CAD build for the part. Positions are in the model's coordinates, mm. A direction names the side the tool comes from. Give positions to 0.01 mm unless a question says otherwise; leave off trailing zeros. Write each loop counter-clockwise with the first axis right and the second up, starting at its lowest first coordinate (ties: lowest second). Pieces come first, ordered by that corner, then holes. Notation, with made-up numbers: (-20.75, 31) -> (4.25, 31) arc R28 ccw to (4.25, 53) -> close; hole circle Ø2 at (34, 43). An arc over 180 degrees is marked (long way). Answer as a JSON object with one key per item and string values.
Autodesk Inventor part; units mm, degrees
ref_plane "YZ Plane" through (0, 0, 0) normal (1, 0, 0) x (0, 1, 0)
ref_plane "XZ Plane" through (0, 0, 0) normal (0, 1, 0) x (-1, 0, 0)
ref_plane "XY Plane" through (0, 0, 0) normal (0, 0, 1) x (1, 0, 0)
sketch "Sketch1" plane through (0, 0, 0) normal (0, 0, 1) x (1, 0, 0)
  arc A0 (-12.6, 10.95) -> (-15.1, 8.45) centre (-12.6, 8.45) ccw
  line L0 (-15.1, 8.45) -> (-15.1, -8.45)
  arc A1 (-15.1, -8.45) -> (-12.6, -10.95) centre (-12.6, -8.45) ccw
  line L1 (-12.6, -10.95) -> (12.6, -10.95)
  arc A2 (12.6, -10.95) -> (15.1, -8.45) centre (12.6, -8.45) ccw
  line L2 (15.1, -8.45) -> (15.1, 8.45)
  arc A3 (15.1, 8.45) -> (12.6, 10.95) centre (12.6, 8.45) ccw
  line L3 (12.6, 10.95) -> (-12.6, 10.95)
  circle A4 centre (11.825, 7.675) radius 1.575
  circle A5 centre (11.825, -7.675) radius 1.575
  line L4 (15.7, 8.45) -> (15.7, -8.45)
  arc A6 (12.6, -11.55) -> (15.7, -8.45) centre (12.6, -8.45) ccw
  line L5 (12.6, -11.55) -> (-12.6, -11.55)
  arc A7 (-15.7, -8.45) -> (-12.6, -11.55) centre (-12.6, -8.45) ccw
  line L6 (-15.7, -8.45) -> (-15.7, 8.45)
  arc A8 (-12.6, 11.55) -> (-15.7, 8.45) centre (-12.6, 8.45) ccw
  line L7 (-12.6, 11.55) -> (12.6, 11.55)
  arc A9 (15.7, 8.45) -> (12.6, 11.55) centre (12.6, 8.45) ccw
  line L8 (19.7, -8.45) -> (19.7, 8.45)
  arc A10 (19.7, 8.45) -> (12.6, 15.55) centre (12.6, 8.45) ccw
  line L9 (12.6, 15.55) -> (-12.6, 15.55)
  arc A11 (-12.6, 15.55) -> (-19.7, 8.45) centre (-12.6, 8.45) ccw
  line L10 (-19.7, 8.45) -> (-19.7, -8.45)
  arc A12 (-19.7, -8.45) -> (-12.6, -15.55) centre (-12.6, -8.45) ccw
  line L11 (-12.6, -15.55) -> (12.6, -15.55)
  arc A13 (12.6, -15.55) -> (19.7, -8.45) centre (12.6, -8.45) ccw
  point P0 (0, 0)
  dimension "d0" = 0.6
  dimension "d1" = 4
extrude "Extrusion1" add sketch "Sketch1" along normal blind 5 contours L3 A3 L2 A2 L1 A1 L0 A0 | A4 | A5 | L4 A6 L5 A7 L6 A8 L7 A9 | A13 L11 A12 L10 A11 L9 A10 L8
sketch "Sketch2" plane through (0, 0, 0) normal (0, 0, -1) x (-1, 0, 0)
  line L0 (12.6, 11.55) -> (-12.6, 11.55)
  arc A0 (15.7, 8.45) -> (12.6, 11.55) centre (12.6, 8.45) ccw
  line L1 (15.7, -8.45) -> (15.7, 8.45)
  arc A1 (12.6, -11.55) -> (15.7, -8.45) centre (12.6, -8.45) ccw
  line L2 (12.6, -10.95) -> (-12.6, -10.95)
  arc A2 (-15.7, -8.45) -> (-12.6, -11.55) centre (-12.6, -8.45) ccw
  line L3 (-15.7, 8.45) -> (-15.7, -8.45)
  arc A3 (-12.6, 11.55) -> (-15.7, 8.45) centre (-12.6, 8.45) ccw
  arc A4 (-12.6, 15.55) -> (-19.7, 8.45) centre (-12.6, 8.45) ccw
  line L4 (-19.7, -8.45) -> (-19.7, 8.45)
  arc A5 (-19.7, -8.45) -> (-12.6, -15.55) centre (-12.6, -8.45) ccw
  line L5 (12.6, -15.55) -> (-12.6, -15.55)
  arc A6 (12.6, -15.55) -> (19.7, -8.45) centre (12.6, -8.45) ccw
  line L6 (19.7, 8.45) -> (19.7, -8.45)
  arc A7 (19.7, 8.45) -> (12.6, 15.55) centre (12.6, 8.45) ccw
  line L7 (-12.6, 15.55) -> (12.6, 15.55)
  line L8 (7.1, -5) -> (15.1, -5)
  line L9 (15.1, -5) -> (15.1, 5)
  line L10 (15.1, 5) -> (7.1, 5)
  line L11 (7.1, 5) -> (7.1, -5)
  line L12 (15.7, 7) -> (19.7, 7)
  line L13 (19.7, 7) -> (19.7, -7)
  line L14 (19.7, -7) -> (15.7, -7)
  line L15 (15.7, -7) -> (15.7, 7)
  line L16 (15.7, 7) -> (19.7, -7) construction
  line L17 (19.7, 7) -> (15.7, -7) construction
  line L18 (-12.6, -11.55) -> (12.6, -11.55)
  point P0 (0, 0)
  point P1 (17.7, 0)
  point P2 (19.7, 0)
  point P3 (17.7, 7)
  dimension "d4" = 2
extrude "Extrusion2" add sketch "Sketch2" along normal blind 9.8 contours L0 A3 L3 A2 L18 A1 L1 L14 L6 A6 L5 A5 L4 A4 L7 A7 L12 A0
sketch "Sketch3" plane through (0, 0, 0) normal (0, 0, -1) x (-1, 0, 0)
  circle A0 centre (-11.825, -7.675) radius 1.575
  circle A1 centre (-11.825, 7.675) radius 1.575
  circle A2 centre (-11.825, -7.675) radius 1.2
  circle A3 centre (-11.825, 7.675) radius 1.2
  point P0 (0, 0)
  dimension "d7" = 3.15
  dimension "d8" = 2.4
  dimension "d9" = 2.4
extrude "Extrusion3" cut sketch "Sketch3" against normal blind 3 contours A2 | A3
sketch "Sketch4" plane through (0, 0, 5) normal (0, 0, 1) x (1, 0, 0)
  arc A0 (19.7, 8.45) -> (12.6, 15.55) centre (12.6, 8.45) ccw
  line L0 (12.6, 15.55) -> (-12.6, 15.55)
  arc A1 (-12.6, 15.55) -> (-19.7, 8.45) centre (-12.6, 8.45) ccw
  line L1 (-19.7, 8.45) -> (-19.7, -8.45)
  arc A2 (-19.7, -8.45) -> (-12.6, -15.55) centre (-12.6, -8.45) ccw
  line L2 (-12.6, -15.55) -> (12.6, -15.55)
  arc A3 (12.6, -15.55) -> (19.7, -8.45) centre (12.6, -8.45) ccw
  line L3 (19.7, -8.45) -> (19.7, 8.45)
  line L4 (-2.6, -15.55) -> (-12.6, -15.55)
  line L5 (-12.6, -15.55) -> (-12.6, -25.55)
  line L6 (-12.6, -25.55) -> (-2.6, -25.55)
  line L7 (-2.6, -25.55) -> (-2.6, -15.55)
  line L8 (-2.6, -15.55) -> (-12.6, -25.55) construction
  line L9 (-12.6, -15.55) -> (-2.6, -25.55) construction
  line L10 (-12.6, -15.55) -> (12.6, -15.55)
  line L11 (19.7, 0) -> (-19.7, 0)
  line L12 (0, 15.55) -> (0, -15.55)
  line L13 (-2.6, 15.55) -> (-12.6, 15.55)
  line L14 (-12.6, 15.55) -> (-12.6, 25.55)
  line L15 (-12.6, 25.55) -> (-2.6, 25.55)
  line L16 (-2.6, 25.55) -> (-2.6, 15.55)
  line L17 (-2.6, 15.55) -> (-12.6, 25.55) construction
  line L18 (-12.6, 15.55) -> (-2.6, 25.55) construction
  arc A4 (19.7, 8.45) -> (12.6, 15.55) centre (12.6, 8.45) ccw
  line L19 (2.6, 15.55) -> (12.6, 15.55)
  line L20 (2.6, 25.55) -> (2.6, 15.55)
  line L21 (2.6, 15.55) -> (12.6, 25.55) construction
  line L22 (12.6, 25.55) -> (2.6, 25.55)
  line L23 (12.6, 15.55) -> (2.6, 25.55) construction
  line L24 (12.6, 15.55) -> (12.6, 25.55)
  line L25 (2.6, -15.55) -> (12.6, -15.55)
  line L26 (2.6, -25.55) -> (2.6, -15.55)
  line L27 (2.6, -15.55) -> (12.6, -25.55) construction
  line L28 (12.6, -15.55) -> (2.6, -25.55) construction
  line L29 (12.6, -15.55) -> (12.6, -25.55)
  line L30 (12.6, -25.55) -> (2.6, -25.55)
  point P0 (0, 0)
  point P1 (-7.6, -20.55)
  point P2 (-7.6, 20.55)
  point P3 (7.6, 20.55)
  point P4 (2.6, 15.55)
  point P5 (-2.6, 15.55)
  point P6 (7.6, -20.55)
  point P7 (2.6, -15.55)
  dimension "d12" = 10
  dimension "d13" = 10
extrude "Extrusion4" add sketch "Sketch4" against normal blind 11 contours L0 L20 L22 L24 | L29 L30 L26 L2
sketch "Sketch5" plane through (0, 0, -6) normal (0, 0, -1) x (-1, 0, 0)
  line L0 (-12.6, -15.55) -> (-2.6, -15.55)
  line L1 (5.6, -22.55) -> (12.6, -15.55)
  line L2 (4.1, -17.05) -> (11.1, -24.05)
  line L3 (12.6, -11.55) -> (-12.6, -11.55)
  arc A0 (-15.7, -8.45) -> (-12.6, -11.55) centre (-12.6, -8.45) ccw
  line L4 (-15.7, -8.45) -> (-15.7, 8.45)
  arc A1 (-12.6, 11.55) -> (-15.7, 8.45) centre (-12.6, 8.45) ccw
  line L5 (-12.6, 11.55) -> (12.6, 11.55)
  arc A2 (15.7, 8.45) -> (12.6, 11.55) centre (12.6, 8.45) ccw
  line L6 (15.7, 8.45) -> (15.7, 7)
  line L7 (15.7, 7) -> (19.7, 7)
  line L8 (19.7, 7) -> (19.7, 8.45)
  arc A3 (19.7, 8.45) -> (12.6, 15.55) centre (12.6, 8.45) ccw
  line L9 (12.6, 15.55) -> (-12.6, 15.55)
  arc A4 (-12.6, 15.55) -> (-19.7, 8.45) centre (-12.6, 8.45) ccw
  line L10 (-19.7, 8.45) -> (-19.7, -8.45)
  arc A5 (-19.7, -8.45) -> (-12.6, -15.55) centre (-12.6, -8.45) ccw
  line L11 (-12.6, -15.55) -> (12.6, -15.55)
  arc A6 (12.6, -15.55) -> (19.7, -8.45) centre (12.6, -8.45) ccw
  line L12 (19.7, -8.45) -> (19.7, -7)
  line L13 (19.7, -7) -> (15.7, -7)
  line L14 (15.7, -7) -> (15.7, -8.45)
  arc A7 (12.6, -11.55) -> (15.7, -8.45) centre (12.6, -8.45) ccw
  circle A8 centre (-11.825, 7.675) radius 1.2
  circle A9 centre (-11.825, -7.675) radius 1.2
  line L15 (19.7, 7) -> (15.7, 7)
  line L16 (15.7, 7) -> (15.7, 8.45)
  arc A10 (15.7, 8.45) -> (12.6, 11.55) centre (12.6, 8.45) ccw
  line L17 (12.6, 11.55) -> (-12.6, 11.55)
  arc A11 (-12.6, 11.55) -> (-15.7, 8.45) centre (-12.6, 8.45) ccw
  line L18 (-15.7, 8.45) -> (-15.7, -8.45)
  arc A12 (-15.7, -8.45) -> (-12.6, -11.55) centre (-12.6, -8.45) ccw
  line L19 (-12.6, -11.55) -> (12.6, -11.55)
  arc A13 (12.6, -11.55) -> (15.7, -8.45) centre (12.6, -8.45) ccw
  line L20 (15.7, -8.45) -> (15.7, -7)
  line L21 (15.7, -7) -> (19.7, -7)
  line L22 (19.7, 7) -> (19.7, -7)
  line L23 (19.7, 0) -> (-19.7, 0)
  line L24 (0, -15.55) -> (0, 15.55)
  line L25 (-12.6, -15.55) -> (-12.6, -25.55)
  line L26 (-12.6, -25.55) -> (-2.6, -25.55)
  line L27 (-2.6, -25.55) -> (-2.6, -15.55)
  point P0 (0, 0)
  point P1 (7.6, -20.55)
  point P2 (7.6, 20.55)
  point P3 (-7.6, 20.55)
  point P4 (-7.6, -20.55)
hole "Hole1" at (7.6, 20.55, -6) at (7.6, -20.55, -6) direction (0, 0, 1) diameter 4.5 end through all
fillet "Fillet1" radius 1 2 edges at (12.6, -15.55, -0.5) (12.6, 15.55, -0.5)
fillet "Fillet2" radius 1 6 edges at (2.6, -15.55, -0.5) (2.6, 15.55, -0.5) (12.6, 25.55, -0.5) (2.6, 25.55, -0.5) (2.6, -25.55, -0.5) (12.6, -25.55, -0.5)
sketch "Sketch6" plane through (0, 0, -9.8) normal (0, 0, -1) x (-1, 0, 0)
  line L0 (12.6, -11.55) -> (-12.6, -11.55)
  arc A0 (-15.7, -8.45) -> (-12.6, -11.55) centre (-12.6, -8.45) ccw
  line L1 (-15.7, -8.45) -> (-15.7, 8.45)
  arc A1 (-12.6, 11.55) -> (-15.7, 8.45) centre (-12.6, 8.45) ccw
  line L2 (-12.6, 11.55) -> (12.6, 11.55)
  arc A2 (15.7, 8.45) -> (12.6, 11.55) centre (12.6, 8.45) ccw
  line L3 (15.7, 8.45) -> (15.7, 7)
  line L4 (15.7, 7) -> (19.7, 7)
  line L5 (19.7, 7) -> (19.7, 8.45)
  arc A3 (19.7, 8.45) -> (12.6, 15.55) centre (12.6, 8.45) ccw
  line L6 (12.6, 15.55) -> (-13.2535, 15.55)
  arc A4 (-13.4765, 15.4957) -> (-13.2535, 15.55) centre (-13.6, 16.488) ccw
  arc A5 (-13.4765, 15.4957) -> (-19.7, 8.45) centre (-12.6, 8.45) ccw
  line L7 (-19.7, 8.45) -> (-19.7, -8.45)
  arc A6 (-19.7, -8.45) -> (-13.4765, -15.4957) centre (-12.6, -8.45) ccw
  arc A7 (-13.2535, -15.55) -> (-13.4765, -15.4957) centre (-13.6, -16.488) ccw
  line L8 (-13.2535, -15.55) -> (12.6, -15.55)
  arc A8 (12.6, -15.55) -> (19.7, -8.45) centre (12.6, -8.45) ccw
  line L9 (19.7, -8.45) -> (19.7, -7)
  line L10 (19.7, -7) -> (15.7, -7)
  line L11 (15.7, -7) -> (15.7, -8.45)
  arc A9 (12.6, -11.55) -> (15.7, -8.45) centre (12.6, -8.45) ccw
  arc A10 (-12.6, 15.55) -> (-19.7, 8.45) centre (-12.6, 8.45) ccw
  arc A11 (-19.7, -8.45) -> (-12.6, -15.55) centre (-12.6, -8.45) ccw
  point P0 (0, 0)
extrude "Extrusion5" cut sketch "Sketch6" against normal up to surface (3.8 mm away) contours L8 A7 A11 | A4 L6 A10
equation "\"d9\" = d8"
properties part number "PrzyciskSTOP_1_3DPrint"
1) Wall check: probe 1 along Y at (x, z) = (7.6, 3.25); probe 2 along Y at (x, z) = (7.6, -1.5); probe 3 along X at (y, z) = (-20.55, -1.25). Give the ranges that are in metal, low to high.
Model answer:
{"probe 1": "y = -25.55 to -22.8, -18.3 to 18.3, 22.8 to 25.55", "probe 2": "y = -25.55 to -22.8, -18.3 to -11.55, 11.55 to 18.3, 22.8 to 25.55", "probe 3": "x = 2.6 to 5.35, 9.85 to 12.6"}
2) Pin check, flat tips, straight feed: pin 1 (5 mm diameter, centred on x = -5.5, y = 20, fed in from -Z); pin 2 (3 mm diameter, centred on y = 12, z = 3, fed in from -X); pin 3 (1.5 mm diameter, centred on x = -12.5, y = 5.5, fed in from -Z); pin 4 (3 mm diameter, centred on y = -17.5, z = -1.5, fed in from -X). Stop position of each tip, or through.
Model answer:
{"pin 1": "passes through", "pin 2": "stops at x = -19.4", "pin 3": "stops at z = 0", "pin 4": "stops at x = 2.44"}
3) Mould opens along Y. For faces 1 (the flat face through (-3, 15.55, -4)), 2 (the flat face through (2.6, 21, 0)), 3 (the flat face through (-15.7, 8, -5)) say: released by +Y, released by -Y, zero draft, split by the parting line, or undercut.
Model answer:
{"face 1": "released by +Y", "face 2": "zero draft", "face 3": "undercut"}
4) Slice it at C-C (x = -1). List the corners of the cut face in (y, z).
Model answer:
{"outline": "(-15.55, -9.8) -> (-11.55, -9.8) -> (-11.55, 0) -> (11.55, 0) -> (11.55, -9.8) -> (15.55, -9.8) -> (15.55, 5) -> (-15.55, 5) -> close"}
5) Slice it at B-B (y = -20.55). List the corners of the cut face in (x, z), then the cut area to 3 significant figures.
Model answer:
{"outline": "(2.6, -6) -> (5.35, -6) -> (5.35, 5) -> (2.6, 5) -> close; (9.85, -6) -> (12.6, -6) -> (12.6, 5) -> (9.85, 5) -> close", "area": "60.5 mm2"}
6) Slice it at D-D (z = 1). List the corners of the cut face in (x, y) (3 decimals).
Model answer:
{"outline": "(-19.7, -8.45) arc R7.1 ccw to (-12.6, -15.55) -> (1.6, -15.55) arc R1 cw to (2.6, -16.55) -> (2.6, -24.55) arc R1 ccw to (3.6, -25.55) -> (11.6, -25.55) arc R1 ccw to (12.6, -24.55) -> (12.6, -16.488) arc R1 cw to (13.477, -15.496) arc R7.1 ccw to (19.7, -8.45) -> (19.7, 8.45) arc R7.1 ccw to (13.477, 15.496) arc R1 cw to (12.6, 16.488) -> (12.6, 24.55) arc R1 ccw to (11.6, 25.55) -> (3.6, 25.55) arc R1 ccw to (2.6, 24.55) -> (2.6, 16.55) arc R1 cw to (1.6, 15.55) -> (-12.6, 15.55) arc R7.1 ccw to (-19.7, 8.45) -> close; hole circle Ø4.5 at (7.6, -20.55); hole circle Ø4.5 at (7.6, 20.55); hole circle Ø2.4 at (11.825, -7.675); hole circle Ø2.4 at (11.825, 7.675)"}
7) Slice it at A-A (x = 7.6). List the corners of the cut face in (y, z).
Model answer:
{"outline": "(-25.55, -6) -> (-22.8, -6) -> (-22.8, 5) -> (-25.55, 5) -> close; (-18.3, -6) -> (-15.55, -6) -> (-15.55, -9.8) -> (-11.55, -9.8) -> (-11.55, 0) -> (11.55, 0) -> (11.55, -9.8) -> (15.55, -9.8) -> (15.55, -6) -> (18.3, -6) -> (18.3, 5) -> (-18.3, 5) -> close; (22.8, -6) -> (25.55, -6) -> (25.55, 5) -> (22.8, 5) -> close"}
8) 3-axis set-ups, long thin cutter, end or side, ignore diameter. For faces 4 (the cylindrical face through (-17.68, -13.41, -2.3)), 5 (the flat face through (-18, -7, -5)), 6 (the cylindrical face through (10.717, -8.135, 1.479)), 7 (the flat face through (12.6, -20, 0)), 8 (the flat face through (7, 23, -6)): which of +Z, -Z, +X, -X, +Y, -Y reach the whole face in a straight line?
Model answer:
{"face 4": "+Z, -Z, -X, -Y", "face 5": "-Z, -X", "face 6": "-Z", "face 7": "+Z, -Z, +X, -Y", "face 8": "-Z, +X, -X, +Y"}
